```python
from build123d import *

# Parameters (mm, degrees)
CROQUIS1_W              = 100
CROQUIS1_H              = 115
CROQUIS1_R              = 4.5
CROQUIS1_W_2            = 14.7
CROQUIS1_H_2            = 2.8
CROQUIS1_W_3            = 22.05
CROQUIS1_H_3            = 3
CROQUIS1_W_4            = 13.85
CROQUIS1_W_5            = 23.75
SALIENTE_EXTRUIR1_DEPTH = 3
CROQUIS2_W              = 35
CROQUIS2_H              = 115
CORTAR_EXTRUIR1_DEPTH   = 4


with BuildPart() as part:
    # Croquis1 → Saliente-Extruir1 (new body)
    with BuildSketch(Plane.XY):
        Rectangle(CROQUIS1_W, CROQUIS1_H)
        with Locations((0, -22.5)):
            Circle(CROQUIS1_R, mode=Mode.SUBTRACT)
        with Locations((-22.9, -22.5)):
            Circle(CROQUIS1_R, mode=Mode.SUBTRACT)
        with Locations((24.1, -22.5)):
            Circle(CROQUIS1_R, mode=Mode.SUBTRACT)
        with Locations((29.95, -46.1)):
            Rectangle(CROQUIS1_W_2, CROQUIS1_H_2, mode=Mode.SUBTRACT)
        with Locations((-29.95, -46.1)):
            Rectangle(CROQUIS1_W_2, CROQUIS1_H_2, mode=Mode.SUBTRACT)
        with Locations((-0.425, -46)):
            Rectangle(CROQUIS1_W_3, CROQUIS1_H_3, mode=Mode.SUBTRACT)
        with Locations((30.375, 52.1)):
            Rectangle(CROQUIS1_W_4, CROQUIS1_H_2, mode=Mode.SUBTRACT)
        with Locations((-30.375, 52.1)):
            Rectangle(CROQUIS1_W_4, CROQUIS1_H_2, mode=Mode.SUBTRACT)
        with Locations((-0.425, 52)):
            Rectangle(CROQUIS1_W_5, CROQUIS1_H_3, mode=Mode.SUBTRACT)
    extrude(amount=SALIENTE_EXTRUIR1_DEPTH)

    # Croquis2 → Cortar-Extruir1 (cut, through all)
    with BuildSketch(Plane.XY.offset(3)):
        with Locations((32.5, 0)):
            Rectangle(CROQUIS2_W, CROQUIS2_H)
    extrude(amount=-CORTAR_EXTRUIR1_DEPTH, mode=Mode.SUBTRACT)


solid = part.part
```
Input: part model. Units: mm. Frame: model coordinates. A direction names the side the tool comes from. Round coordinates to 2 decimals unless told otherwise and drop trailing zeros. Order: outer loops, then holes, each group sorted by start corner. A loop starts at its lowest first (then second) coordinate and runs counter-clockwise, first axis right, second up. Notation, with made-up numbers: (-25, -17.75) - (-13, -17.75) arc R19 ccw to (-13, 15.25) - close; hole circle Ø4 at (56, -28.5). An arc over 180 degrees is marked (long way). Answer in a Markdown table with one row per item.
Item 1: Section query B-B (x = 0). Return the cut outline in (y, z).
Model answer:
| item | result |
|---|---|
| outline | (-57.5, 0) - (-47.5, 0) - (-47.5, 3) - (-57.5, 3) - close; (-44.5, 0) - (-27, 0) - (-27, 3) - (-44.5, 3) - close; (-18, 0) - (50.5, 0) - (50.5, 3) - (-18, 3) - close; (53.5, 0) - (57.5, 0) - (57.5, 3) - (53.5, 3) - close |
Item 2: Pin query (flat end, axial travel): pin 1 (7 mm diameter, centred on x = -22.9, y = -22.5, fed in from -Z). Return the tip coordinate at first contact, or that it passes through.
Model answer:
| item | result |
|---|---|
| pin 1 | passes through |
Item 3: Mould query, pull axis X, two halves, no side actions, for faces 3 (the flat face through (-30, -47.5, 1)), 4 (the flat face through (-18, 1, 3)), 5 (the flat face through (15, -1, 2)). Classes: released by +X, released by -X, zero draft, split by the parting line, or undercut.
Model answer:
| item | result |
|---|---|
| face 3 | undercut |
| face 4 | zero draft |
| face 5 | released by +X |
Item 4: Reachability of faces 1 (the flat face through (11.45, 52, 1)), 2 (the flat face through (-18, 57.5, 1)) from +Z, -Z, +X, -X, +Y, -Y: full face, straight path, thin tool, end or side. Return the list, or none.
Model answer:
| item | result |
|---|---|
| face 1 | +Z, -Z |
| face 2 | +Z, -Z, +X, -X, +Y |
Item 5: Line query: line 1 (Y direction, x = -30.5, z = 0.45); line 2 (Y direction, x = 0, z = 2.25); line 3 (Y direction, x = -22.9, z = 2.25). Output: solid intervals per line, ascending.
Model answer:
| item | result |
|---|---|
| line 1 | y = -57.5 to -47.5, -44.7 to 50.7, 53.5 to 57.5 |
| line 2 | y = -57.5 to -47.5, -44.5 to -27, -18 to 50.5, 53.5 to 57.5 |
| line 3 | y = -57.5 to -47.5, -44.7 to -27, -18 to 57.5 |
Item 6: Section query D-D (x = -21). Return the cut outline in (y, z), then the cut area to 3 significant figures.
Model answer:
| item | result |
|---|---|
| outline | (-57.5, 0) - (-26.58, 0) - (-26.58, 3) - (-57.5, 3) - close; (-18.42, 0) - (57.5, 0) - (57.5, 3) - (-18.42, 3) - close |
| area | 321 mm² |
Item 7: Section query A-A (y = -22.5). Return the cut outline in (x, z), then the cut area to 3 significant figures.
Model answer:
| item | result |
|---|---|
| outline | (-50, 0) - (-27.4, 0) - (-27.4, 3) - (-50, 3) - close; (-18.4, 0) - (-4.5, 0) - (-4.5, 3) - (-18.4, 3) - close; (4.5, 0) - (15, 0) - (15, 3) - (4.5, 3) - close |
| area | 141 mm² |
Item 8: Section query C-C (z = 1.2). Return the cut outline in (x, y), then the cut area to 3 significant figures.
Model answer:
| item | result |
|---|---|
| outline | (-50, -57.5) - (15, -57.5) - (15, 57.5) - (-50, 57.5) - close; hole (-37.3, -47.5) - (-22.6, -47.5) - (-22.6, -44.7) - (-37.3, -44.7) - close; hole (-37.3, 50.7) - (-23.45, 50.7) - (-23.45, 53.5) - (-37.3, 53.5) - close; hole circle Ø9 at (-22.9, -22.5); hole (-12.3, 50.5) - (11.45, 50.5) - (11.45, 53.5) - (-12.3, 53.5) - close; hole (-11.45, -47.5) - (10.6, -47.5) - (10.6, -44.5) - (-11.45, -44.5) - close; hole circle Ø9 at (0, -22.5) |
| area | 7,130 mm² |
